from build123d import *

# Parameters (mm, degrees)
F0_W      = 45.5
F0_H      = 2
F1_DEPTH  = 35
F0_H_2    = 43
F0_R      = 1.75
F0_R_2    = 11.5
F2_DEPTH  = 6.6
F0_W_2    = 6.35
F0_H_3    = 8.8
F3_DEPTH  = 6.6
F4_R      = 2
F5_DEPTH  = 14
F6_W      = 5
F6_H      = 8.3
F7_DEPTH  = 8.39
F8_SIZE2  = 28.4
F8_SIZE   = 45.5
F9_R      = 2
F10_SIZE  = 1
F11_SIZE  = 4
F12_SIZE  = 5
F13_W     = 22.4
F13_H     = 37
F14_DEPTH = 8
F15_SIZE  = 7.99999
F16_SIZE  = 2


# Not quite as in the source:
# - a fillet or chamfer is up to 0.001 mm smaller than in the source, because OpenCascade refuses the exact size


with BuildPart() as f1:
    # F0 (on Right) → F1 (new body)
    with BuildSketch(Plane.YZ):
        Polygon((35, 21.5), (24, 21.5), (24, -21.5), (24, -23.5), (35, -23.5), (35, -17.88), (35, -9.08), (35, 5.92), (35, 14.72), align=None)
        with Locations((1.25, -22.5)):
            Rectangle(F0_W, F0_H)
    extrude(amount=F1_DEPTH)

    # F0 (on Right) → F2 (join)
    with BuildSketch(Plane.YZ):
        with Locations((1.25, 0)):
            Rectangle(F0_W, F0_H_2)
        with Locations((-15.5, -15.5)):
            Circle(F0_R, mode=Mode.SUBTRACT)
        with Locations((15.5, -15.5)):
            Circle(F0_R, mode=Mode.SUBTRACT)
        Circle(F0_R_2, mode=Mode.SUBTRACT)
        with Locations((-15.5, 15.5)):
            Circle(F0_R, mode=Mode.SUBTRACT)
        with Locations((15.5, 15.5)):
            Circle(F0_R, mode=Mode.SUBTRACT)
    extrude(amount=F2_DEPTH)

    # F0 (on Right) → F3 (join)
    with BuildSketch(Plane.YZ):
        with Locations((38.175, 10.32)):
            Rectangle(F0_W_2, F0_H_3)
        with Locations((38.175, -13.48)):
            Rectangle(F0_W_2, F0_H_3)
    extrude(amount=F3_DEPTH)

    # F4 (on face) → F5 (cut)
    with BuildSketch(Plane(origin=(0, 35, 0), x_dir=(-1, 0, 0), z_dir=(0, 1, 0))):
        with Locations((-3.3, -1.58)):
            Circle(F4_R)
    extrude(amount=-F5_DEPTH, mode=Mode.SUBTRACT)

    # F6 (on face) → F7 (cut)
    with BuildSketch(Plane(origin=(0, 0, 0), x_dir=(0, -1, 0), z_dir=(-1, 0, 0))):
        with Locations((-27.5, -1.58)):
            Rectangle(F6_W, F6_H)
    extrude(amount=-F7_DEPTH, mode=Mode.SUBTRACT)

    # F8
    f8_edges = [f1.edges().sort_by_distance(p)[0] for p in [
        (35, -21.5, -22.5),
    ]]
    f8_side = f1.faces().sort_by_distance((35, 25.113055, -4.338737))[0]
    chamfer(f8_edges, length=F8_SIZE, length2=F8_SIZE2, reference=f8_side)

    # F9
    f9_edges = [f1.edges().sort_by_distance(p)[0] for p in [
        (3.3, 41.35, 14.72),
        (3.3, 41.35, 5.92),
        (3.3, 41.35, -9.08),
        (3.3, 41.35, -17.88),
    ]]
    fillet(f9_edges, radius=F9_R)

    # F10
    f10_edges = [f1.edges().sort_by_distance(p)[0] for p in [
        (0, 37.175, -9.08),
        (0, 37.175, 14.72),
        (6.6, 37.175, -17.88),
        (6.6, 37.175, 5.92),
    ]]
    chamfer(f10_edges, length=F10_SIZE)

    # F11
    f11_edges = [f1.edges().sort_by_distance(p)[0] for p in [
        (3.3, -21.5, 21.5),
    ]]
    chamfer(f11_edges, length=F11_SIZE)

    # F12
    f12_edges = [f1.edges().sort_by_distance(p)[0] for p in [
        (0, -11.5, 0),
    ]]
    chamfer(f12_edges, length=F12_SIZE)

    # F13 (on face) → F14 (cut)
    with BuildSketch(Plane.XZ.offset(-24)):
        with Locations((20.8, 0)):
            Rectangle(F13_W, F13_H)
    extrude(amount=-F14_DEPTH, mode=Mode.SUBTRACT)

    # F15 (size 8 in the source; OpenCascade refuses exactly that, so slightly less here)
    f15_edges = [f1.edges().sort_by_distance(p)[0] for p in [
        (20.8, 32, 18.5),
        (9.6, 32, 0),
        (20.8, 32, -18.5),
        (32, 32, 0),
    ]]
    chamfer(f15_edges, length=F15_SIZE)

    # F16
    f16_edges = [f1.edges().sort_by_distance(p)[0] for p in [
        (35, 29.5, 21.5),
    ]]
    chamfer(f16_edges, length=F16_SIZE)


solid = f1.part
Source: CAD feature listing. Evaluate the final solid. Frame: model axes, mm. A direction names the side the tool comes from. Coordinates: 2 decimals unless noted, no trailing zeros. Loops run counter-clockwise (first coordinate to the right, second up) from the corner with the lowest first, then second, coordinate; pieces in that order, holes last. Notation, with made-up numbers: (32.25, 70.25) -> (63.25, 70.25) arc R32 cw to (63.25, 109.25) -> close; hole circle Ø2 at (3, 77.25). An arc over 180 degrees is marked (long way). Answer in a Markdown table with one row per item. Add a question column.
Q1. Reachability of faces 4 (the face through (3, 37, 5.92)), 5 (the face through (4, 28, 2.57)), 6 (the face through (28, 28, 0)) from +Z, -Z, +X, -X, +Y, -Y: full face, straight path, thin tool, end or side. Return the list, or none.
Q2. Section B-B on y = 0. Return the cut outline in (x, z), and give its area (3 significant figures).
Q3. Pull-direction query (Z, two-part tool) for faces 1 (the face through (13, 13, -23.5)), 2 (the face through (20.6, 27.2, -15.3)), 3 (the face through (5, 20, 21.5)); classes: pulls with the +Z half, pulls with the -Z half, needs draft (parallel to the pull), parting line crosses it, or undercut.
Q4. Section A-A on x = 3.3. Give the number of separate pieces and of enclosed holes in the cut face, and give its area (3 significant figures).
Q5. Ray query, line 1 along Z through (x, y) = (2, 15.5); line 2 along X through (y, z) = (0.5, -19); line 3 along Y through (x, z) = (33, 8.5). Return the intervals inside material, ascending.
Q6. Contact query for flat-ended pins moving along their axis: pin 1 Ø6 at (y, z) = (14.5, 10.5) entering from +X; pin 2 Ø2 at (x, y) = (2.5, 36.5) entering from +Z; pin 3 Ø1.2 at (x, z) = (4, -2) entering from +Y. Output: stop coordinate, or through.
Computed values:
| question | item | result |
|---|---|---|
| 1 | face 4 | +X, -X, +Y |
| 1 | face 5 | -X |
| 1 | face 6 | -Y |
| 2 | outline | (0, -23.5) -> (20.02, -23.5) -> (20.02, -21.5) -> (6.6, -21.5) -> (6.6, -11.5) -> (5, -11.5) -> (0, -16.5) -> close; (0, 16.5) -> (5, 11.5) -> (6.6, 11.5) -> (6.6, 21.5) -> (0, 21.5) -> close |
| 2 | area | 147 mm^2 |
| 3 | face 1 | pulls with the -Z half |
| 3 | face 2 | undercut |
| 3 | face 3 | pulls with the +Z half |
| 4 | separate pieces | 1 |
| 4 | enclosed holes | 5 |
| 4 | area | 1,980 mm^2 |
| 5 | line 1 | z = -23.5 to -17.25, -13.75 to 13.75, 17.25 to 21.5 |
| 5 | line 2 | x = 0 to 6.6 |
| 5 | line 3 | y = 24 to 35 |
| 6 | pin 1 | stops at x = 6.6 |
| 6 | pin 2 | stops at z = 14.72 |
| 6 | pin 3 | stops at y = 21 |
